from build123d import *

# Parameters (mm, degrees)
SKETCH_1_R          = 37.83
EXTRUDE_1_DEPTH     = 18.1
DRAFT_1_ANGLE       = -2
SKETCH_3_R          = 34
EXTRUDE_2_DEPTH     = 1.53
SKETCH_4_R          = 37.197934072
EXTRUDE_3_DEPTH     = 22.37
DRAFT_2_ANGLE       = -5
SKETCH_5_R          = 1.5
CUT_EXTRUDE_1_DEPTH = 10
CUT_EXTRUDE_2_DEPTH = 30


with BuildPart() as part:
    # 草图1 → 凸台-拉伸1 (new body)
    with BuildSketch(Plane(origin=(0, 0, 0), x_dir=(1, 0, 0), z_dir=(0, 1, 0))):
        with Locations(Location((0, 0, 0), (0, 0, 90))):
            Circle(SKETCH_1_R)
    extrude(amount=EXTRUDE_1_DEPTH)

    # 拔模1
    draft_1_faces = [part.faces().sort_by_distance(p)[0] for p in [
        (0, 9.05, 37.83),
    ]]
    draft(draft_1_faces, Plane(origin=(0, 0, 0), x_dir=(0, 0, -1), z_dir=(0, -1, 0)), DRAFT_1_ANGLE)

    # 草图3 → 凸台-拉伸2 (add)
    with BuildSketch(Plane(origin=(0, 18.1, 0), x_dir=(1, 0, 0), z_dir=(0, 1, 0))):
        with Locations(Location((0, 0, 0), (0, 0, 270))):
            Circle(SKETCH_3_R)
    extrude(amount=EXTRUDE_2_DEPTH)

    # 草图4 → 凸台-拉伸3 (add)
    with BuildSketch(Plane(origin=(0, 19.63, 0), x_dir=(1, 0, 0), z_dir=(0, 1, 0))):
        with Locations(Location((0, 0, 0), (0, 0, 270))):
            Circle(SKETCH_4_R)
    extrude(amount=EXTRUDE_3_DEPTH)

    # 拔模2
    draft_2_faces = [part.faces().sort_by_distance(p)[0] for p in [
        (0, 30.815, -37.197934072),
    ]]
    draft(draft_2_faces, Plane(origin=(0, 19.63, 0), x_dir=(0, 0, -1), z_dir=(0, -1, 0)), DRAFT_2_ANGLE)

    # 草图5 → 切除-拉伸1 (cut)
    with BuildSketch(Plane.XZ):
        with Locations(Location((29, 0, 0), (0, 0, 270))):
            Circle(SKETCH_5_R)
        with Locations(Location((-29, 0, 0), (0, 0, 90))):
            Circle(SKETCH_5_R)
        with Locations(Location((0, 29, 0), (0, 0, 270))):
            Circle(SKETCH_5_R)
        with Locations(Location((0, -29, 0), (0, 0, 90))):
            Circle(SKETCH_5_R)
    extrude(amount=-CUT_EXTRUDE_1_DEPTH, mode=Mode.SUBTRACT)

    # 草图6 → 切除-拉伸2 (cut)
    with BuildSketch(Plane.XY.offset(40)):
        with BuildLine():
            Line((8, 35), (16, 35))
            ThreePointArc((16, 35), (21, 30), (16, 25))
            Line((16, 25), (8, 25))
            ThreePointArc((8, 25), (3, 30), (8, 35))
        make_face()
        with BuildLine():
            Line((-15, 33), (-9, 33))
            ThreePointArc((-9, 33), (-6, 30), (-9, 27))
            Line((-9, 27), (-15, 27))
            ThreePointArc((-15, 27), (-18, 30), (-15, 33))
        make_face()
    extrude(amount=-CUT_EXTRUDE_2_DEPTH, mode=Mode.SUBTRACT)


solid = part.part
The listing builds one solid part. Answer for the finished solid, in the listing's coordinates (mm). A direction names the side the tool comes from. Coordinates: 2 decimals unless noted, no trailing zeros. Order: outer loops, then holes, each group sorted by start corner. A loop starts at its lowest first (then second) coordinate and runs counter-clockwise, first axis right, second up.
Q1. Given P1, Ø2.5, axis at x = -29, z = 0, coming from the -Y side; P2, Ø5, axis at x = 26.5, y = 28.5, coming from the -Z side; P3, Ø2, axis at x = -9, y = 6.5, coming from the +Z side, each flat-ended and moving along its own axis, determine where each tip first touches the part or whether it passes through.
Q2. A cutting plane is placed at D-D, the plane y = 4.5. Write down the section's boundary in (x, z), and give its area (3 significant figures).
Q3. For a pull along Y with two mould halves and no side action, classify faces 4 (the face through (3, 30, 23)), 5 (the face through (-11.25, 10.93, -35.72)), 6 (the face through (30.487, 4.93, 0.195)) as pulls with the +Y half, pulls with the -Y half, needs draft (parallel to the pull), parting line crosses it, or undercut.
Q4. Consider line 1 (X direction, y = 7, z = 0); line 2 (Y direction, x = -33, z = 9); line 3 (Z direction, x = -29, y = 5.75). Determine where each line is inside the solid, lowest interval first.
Q5. Which of the six approach directions +Z, -Z, +X, -X, +Y, -Y give full straight-line access (tool end or side, diameter ignored) to faces 1 (the face through (-29, 10, 0)), 2 (the face through (-12, 33, 23)), 3 (the face through (30.1, 18.1, -16.4))?
Q6. A cutting plane is placed at C-C, the plane y = 30. Write down the section's boundary in (x, z), and give its area (3 significant figures).
Q7. A cutting plane is placed at A-A, the plane z = 0. Write down the section's boundary in (x, y).
Q8. A cutting plane is placed at B-B, the plane x = 0. Write down the section's boundary in (y, z).
Answers follow:
1. P1: stops at y = 10
1. P2: stops at z = -27.42
1. P3: stops at z = 36.75
2. outline: circle Ø75.35 at (0, 0); hole circle Ø3 at (-29, 0); hole circle Ø3 at (0, -29); hole circle Ø3 at (0, 29); hole circle Ø3 at (29, 0)
2. area: 4,430 mm2
3. face 4: undercut
3. face 5: pulls with the +Y half
3. face 6: needs draft
4. line 1: x = -37.59 to -30.5, -27.5 to 27.5, 30.5 to 37.59
4. line 2: y = 0 to 18.1, 19.63 to 42
4. line 3: z = -23.98 to -1.5, 1.5 to 23.98
5. face 1: -Y
5. face 2: +Z
5. face 3: none
6. outline: (-18, 10) - (-18, 31.51) arc R36.29 ccw (long way) to (21, 29.6) - (21, 10) - (3, 10) - (3, 36.17) arc R36.29 ccw to (-6, 35.79) - (-6, 10) - close
6. area: 3,420 mm2
7. outline: (-37.83, 0) - (-30.5, 0) - (-30.5, 10) - (-27.5, 10) - (-27.5, 0) - (27.5, 0) - (27.5, 10) - (30.5, 10) - (30.5, 0) - (37.83, 0) - (37.2, 18.1) - (34, 18.1) - (34, 19.63) - (37.2, 19.63) - (35.24, 42) - (-35.24, 42) - (-37.2, 19.63) - (-34, 19.63) - (-34, 18.1) - (-37.2, 18.1) - close
8. outline: (0, -37.83) - (18.1, -37.2) - (18.1, -34) - (19.63, -34) - (19.63, -37.2) - (42, -35.24) - (42, 35.24) - (19.63, 37.2) - (19.63, 34) - (18.1, 34) - (18.1, 37.2) - (0, 37.83) - (0, 30.5) - (10, 30.5) - (10, 27.5) - (0, 27.5) - (0, -27.5) - (10, -27.5) - (10, -30.5) - (0, -30.5) - close
